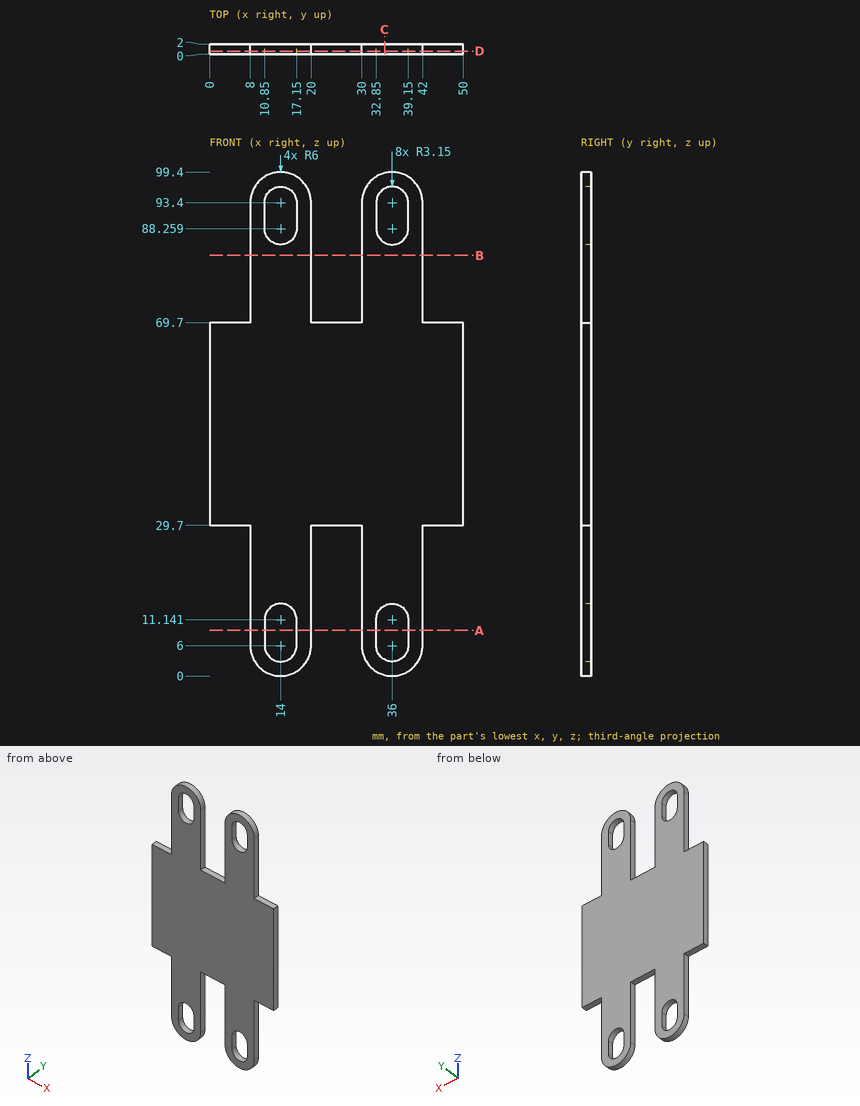
Part print with two shaded views. Sizes in mm from the minimum x, y, z corner. Round coordinates to 2 decimals unless told otherwise and drop trailing zeros. Loops run counter-clockwise (first coordinate to the right, second up) from the corner with the lowest first, then second, coordinate; pieces in that order, holes last. Notation, with made-up numbers: (34, 23.5) - (73, 23.5) arc R23 ccw to (73, 50.5) - close; hole circle Ø4 at (53.25, 85). An arc over 180 degrees is marked (long way). Answer as a JSON object with one key per item and string values.
Item 1: Band-saw the part on A-A on z = 9. List the corners of the cut face in (x, y).
Output:
{"outline": "(8, 0) - (10.85, 0) - (10.85, 2) - (8, 2) - close; (17.15, 0) - (20, 0) - (20, 2) - (17.15, 2) - close; (30, 0) - (32.85, 0) - (32.85, 2) - (30, 2) - close; (39.15, 0) - (42, 0) - (42, 2) - (39.15, 2) - close"}
Item 2: Band-saw the part on B-B on z = 83. List the corners of the cut face in (x, y).
Output:
{"outline": "(8, 0) - (20, 0) - (20, 2) - (8, 2) - close; (30, 0) - (42, 0) - (42, 2) - (30, 2) - close"}
Item 3: Pin check, flat tips, straight feed: pin 1 (0.6 mm diameter, centred on y = 1, z = 87, fed in from +X); pin 2 (1 mm diameter, centred on y = 0.5, z = 12.5, fed in from -X). Stop position of each tip, or through.
Output:
{"pin 1": "x = 42", "pin 2": "x = 8"}
Item 4: Band-saw the part on C-C on x = 34.5. List the corners of the cut face in (y, z), plus the area to 3 significant figures.
Output:
{"outline": "(0, 0.19) - (2, 0.19) - (2, 3.23) - (0, 3.23) - close; (0, 13.91) - (2, 13.91) - (2, 85.49) - (0, 85.49) - close; (0, 96.17) - (2, 96.17) - (2, 99.21) - (0, 99.21) - close", "area": "155 mm2"}
Item 5: Band-saw the part on D-D on y = 0.6. State how many separate pieces and enclosed holes the cut face has, plus the area to 3 significant figures.
Output:
{"separate pieces": "1", "enclosed holes": "4", "area": "3,110 mm2"}
Item 6: Wall check: L1, parallel to X at y = 1.45, z = 80.5; L2, parallel to X at y = 1.9, z = 86.5; L3, parallel to Z at x = 46.5, y = 0.95. Give the ranges that are in metal, low to high.
Output:
{"L1": "8 to 20, 30 to 42", "L2": "8 to 11.39, 16.61 to 20, 30 to 33.39, 38.61 to 42", "L3": "29.7 to 69.7"}
